Can you work these out from the model? Positions are in its coordinate system, mm. Give positions to 0.01 mm unless a question says otherwise; leave off trailing zeros. Order: outer loops, then holes, each group sorted by start corner. A loop starts at its lowest first (then second) coordinate and runs counter-clockwise, first axis right, second up. Notation, with made-up numbers: M -20.5,79 L 35.5,79 A21 cw 35.5,101 Z; hole C 85.5,6.25 d2. An arc over 180 degrees is marked long. One line per question, with ' | ' between items. Start each with the question number.
1) I'm going to push flat-ended pins straight in: pin 1 Ø3 at (y, z) = (1, 1273) entering from -X; pin 2 Ø20 at (x, z) = (663.6, 1242.94) entering from -Y; pin 3 Ø1.5 at (x, y) = (685.5, 3) entering from -Z; pin 4 Ø1.5 at (x, y) = (669, 3) entering from -Z. Where does each tip first touch, or does it pass through?
2) Thinking about a two-plate mould opening in X: for faces 1 (the flat face through (661, 0, 1254)), 2 (the cylindrical face through (681.06, 2.61, 1243.79)), 3 (the cylindrical face through (652.708, 2.613, 1274.831)), which applies, +X half, -X half, draft (parallel to the pull), parting line (faces both ways), or undercut?
3) If we section it at C-C, the plane y = 1.1: State how many separate pieces and enclosed holes the cut face has, plus the area to 3 significant figures.
4) If we section it at A-A, the plane x = 666: Please give me the cut outline in (y, z), plus the area to 3 significant figures.
5) If we section it at D-D, the plane z = 1223: Please give me the cut outline in (x, y), plus the area to 3 significant figures.
6) If we section it at B-B, the plane z = 1252: Please give me the cut outline in (x, y), plus the area to 3 significant figures.
7) Please list where these lines run through material, in increasing order: line 1 along Z through (x, y) = (689, 2.8); line 2 along X through (y, z) = (3.45, 1257.5); line 3 along Z through (x, y) = (687, 1.9). Write a range as [from, to].
```python
from build123d import *

# Parameters (mm, degrees)
SKETCH3_R           = 7.65
SKETCH3_R_2         = 2.15
BOSS_EXTRUDE1_DEPTH = 5.3


with BuildPart() as part:
    # Sketch3 → Boss-Extrude1 (new body)
    with BuildSketch(Plane(origin=(0, 0, 0), x_dir=(1, 0, 0), z_dir=(0, 1, 0))):
        with BuildLine():
            ThreePointArc((653.944459341, -1220.242432272), (637.731714088, -1218.814624577), (636.327920195, -1235.029466732))
            ThreePointArc((636.327920195, -1235.029466732), (637.221930793, -1238.210887622), (635.417200611, -1240.979216142))
            ThreePointArc((635.417200611, -1240.979216142), (630.100805603, -1251.003580625), (635.975748621, -1260.711154148))
            ThreePointArc((635.975748621, -1260.711154148), (637.727498088, -1262.697402891), (637.854371527, -1265.34272204))
            ThreePointArc((637.854371527, -1265.34272204), (639.774817514, -1271.674124807), (646.352289419, -1272.389412948))
            ThreePointArc((646.352289419, -1272.389412948), (648.975379282, -1272.024433719), (651.251559888, -1273.378247634))
            ThreePointArc((651.251559888, -1273.378247634), (652.730141334, -1274.850178419), (654.450327382, -1276.030747471))
            ThreePointArc((654.450327382, -1276.030747471), (656.202076849, -1278.016996214), (656.328950289, -1280.662315363))
            ThreePointArc((656.328950289, -1280.662315363), (658.249396276, -1286.99371813), (664.826868181, -1287.709006271))
            ThreePointArc((664.826868181, -1287.709006271), (667.449958044, -1287.344027042), (669.726138649, -1288.697840957))
            ThreePointArc((669.726138649, -1288.697840957), (685.938883902, -1290.125648653), (687.342677795, -1273.910806497))
            ThreePointArc((687.342677795, -1273.910806497), (686.448667197, -1270.729385607), (688.253397379, -1267.961057087))
            ThreePointArc((688.253397379, -1267.961057087), (693.569792387, -1257.936692604), (687.694849369, -1248.229119081))
            ThreePointArc((687.694849369, -1248.229119081), (685.943099902, -1246.242870338), (685.816226463, -1243.59755119))
            ThreePointArc((685.816226463, -1243.59755119), (683.895780476, -1237.266148422), (677.318308571, -1236.550860281))
            ThreePointArc((677.318308571, -1236.550860281), (674.695218708, -1236.91583951), (672.419038102, -1235.562025595))
            ThreePointArc((672.419038102, -1235.562025595), (670.940456656, -1234.09009481), (669.220270608, -1232.909525758))
            ThreePointArc((669.220270608, -1232.909525758), (667.468521141, -1230.923277015), (667.341647701, -1228.277957867))
            ThreePointArc((667.341647701, -1228.277957867), (665.421201714, -1221.946555099), (658.843729809, -1221.231266958))
            ThreePointArc((658.843729809, -1221.231266958), (656.220639946, -1221.596246187), (653.944459341, -1220.242432272))
        make_face()
        with Locations((645.125239428, -1227.62290381)):
            Circle(SKETCH3_R, mode=Mode.SUBTRACT)
        with Locations((663.599818189, -1242.942497133)):
            Circle(SKETCH3_R, mode=Mode.SUBTRACT)
        with Locations((682.074396951, -1258.262090456)):
            Circle(SKETCH3_R, mode=Mode.SUBTRACT)
        with Locations((678.545358562, -1281.317369419)):
            Circle(SKETCH3_R, mode=Mode.SUBTRACT)
        with Locations((660.070779801, -1265.997776096)):
            Circle(SKETCH3_R, mode=Mode.SUBTRACT)
        with Locations((641.596201039, -1250.678182773)):
            Circle(SKETCH3_R, mode=Mode.SUBTRACT)
        with Locations((643.604715845, -1267.055480116)):
            Circle(SKETCH3_R_2, mode=Mode.SUBTRACT)
        with Locations((662.079294606, -1282.375073439)):
            Circle(SKETCH3_R_2, mode=Mode.SUBTRACT)
        with Locations((680.065882145, -1241.884793113)):
            Circle(SKETCH3_R_2, mode=Mode.SUBTRACT)
        with Locations((661.591303384, -1226.56519979)):
            Circle(SKETCH3_R_2, mode=Mode.SUBTRACT)
    extrude(amount=BOSS_EXTRUDE1_DEPTH)


solid = part.part
```
Results found:
1) pin 1: stops at x = 639.57 | pin 2: stops at y = 0 | pin 3: stops at z = 1238.14 | pin 4: stops at z = 1232.15
2) face 1: draft | face 2: undercut | face 3: -X half
3) separate pieces: 1 | enclosed holes: 10 | area: 1,980 mm²
4) outline: M 0,1222.5 L 5.3,1222.5 L 5.3,1235.68 L 0,1235.68 Z; M 0,1250.21 L 5.3,1250.21 L 5.3,1261.16 L 0,1261.16 Z; M 0,1270.83 L 5.3,1270.83 L 5.3,1287.32 L 0,1287.32 Z | area: 215 mm²
5) outline: M 634.6,0 L 639.03,0 L 639.03,5.3 L 634.6,5.3 Z; M 651.22,0 L 666.42,0 L 666.42,5.3 L 651.22,5.3 Z | area: 104 mm²
6) outline: M 630.17,0 L 634.06,0 L 634.06,5.3 L 630.17,5.3 Z; M 649.13,0 L 677.68,0 L 677.68,5.3 L 649.13,5.3 Z; M 686.47,0 L 691.72,0 L 691.72,5.3 L 686.47,5.3 Z | area: 200 mm²
7) line 1: z = [1249.08, 1255.01], [1261.51, 1267.44], [1276.53, 1286.11] | line 2: x = [632.34, 638.13], [645.06, 674.46], [689.69, 693.55] | line 3: z = [1247.74, 1252.41], [1264.12, 1269.23], [1273.44, 1289.11]
